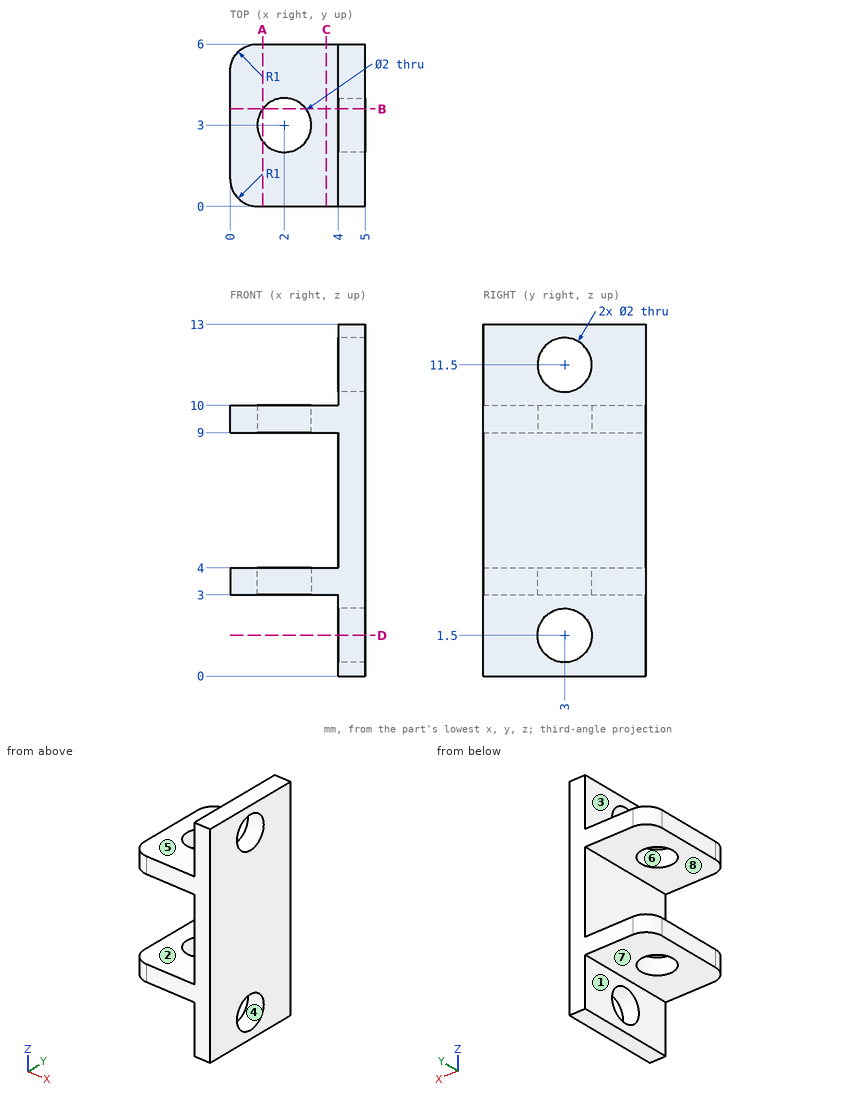
Geometry check sheet. Reference: drawing and pictorial views, mm from the part's lowest x, y, z. A direction names the side the tool comes from. Round coordinates to 2 decimals unless told otherwise and drop trailing zeros. Loops run counter-clockwise (first coordinate to the right, second up) from the corner with the lowest first, then second, coordinate; pieces in that order, holes last. Notation, with made-up numbers: (5, 71) - (23, 71) arc R11 ccw to (23, 76) - close; hole circle Ø1 at (22.25, 75.25). An arc over 180 degrees is marked (long way). Use a Markdown table: item, result. Add a question column.
1. Section check D-D, the plane z = 1.5. Record the boundary of the cut face in (x, y).
2. Release check for a two-part mould opening along Z. For the marked faces 5, 6, 7 and 8 record: released by +Z, released by -Z, zero draft, split by the parting line, or undercut.
3. Gauge pin test, flat ends, axial feed: pin 1 (2.5 mm diameter, centred on y = 2, z = 7, fed in from -X); pin 2 (0.9 mm diameter, centred on y = 3.5, z = 1.5, fed in from -X); pin 3 (2 mm diameter, centred on x = 2, y = 1.5, fed in from +Z); pin 4 (1.2 mm diameter, centred on x = 3, y = 3.5, fed in from -Z). Record the tip position at first contact, or that the pin passes through.
4. Thickness scan on probe 1 along Z at (x, y) = (4.5, 3); probe 2 along Y at (x, z) = (2, 9.8); probe 3 along Z at (x, y) = (0.8, 3.5). Record the ranges inside material, lowest first. Write a range as [from, to].
5. Section check C-C, the plane x = 3.55. Record the boundary of the cut face in (y, z).
6. Section check B-B, the plane y = 3.6. Record the boundary of the cut face in (x, z), plus the area to 3 significant figures.
7. Access from +Z, -Z, +X, -X, +Y, -Y to the whole of each face (thin tool, end or side, straight path). Record for the marked faces 1, 2, 3 and 4.
8. Section check A-A, the plane x = 1.2. Record the boundary of the cut face in (y, z), plus the area to 3 significant figures.
Checks:
| question | item | result |
|---|---|---|
| 1 | outline | (4, 0) - (5, 0) - (5, 2) - (4, 2) - close; (4, 4) - (5, 4) - (5, 6) - (4, 6) - close |
| 2 | face 5 | released by +Z |
| 2 | face 6 | zero draft |
| 2 | face 7 | released by -Z |
| 2 | face 8 | undercut |
| 3 | pin 1 | stops at x = 4 |
| 3 | pin 2 | passes through |
| 3 | pin 3 | stops at z = 10 |
| 3 | pin 4 | stops at z = 3 |
| 4 | probe 1 | z = [0, 0.5], [2.5, 10.5], [12.5, 13] |
| 4 | probe 2 | y = [0, 2], [4, 6] |
| 4 | probe 3 | z = [3, 4], [9, 10] |
| 5 | outline | (0, 3) - (6, 3) - (6, 4) - (0, 4) - close; (0, 9) - (6, 9) - (6, 10) - (0, 10) - close |
| 6 | outline | (0, 3) - (1.2, 3) - (1.2, 4) - (0, 4) - close; (0, 9) - (1.2, 9) - (1.2, 10) - (0, 10) - close; (2.8, 3) - (4, 3) - (4, 2.3) - (5, 2.3) - (5, 10.7) - (4, 10.7) - (4, 10) - (2.8, 10) - (2.8, 9) - (4, 9) - (4, 4) - (2.8, 4) - close; (4, 0) - (5, 0) - (5, 0.7) - (4, 0.7) - close; (4, 12.3) - (5, 12.3) - (5, 13) - (4, 13) - close |
| 6 | area | 14.6 mm^2 |
| 7 | face 1 | -Z, -X, +Y, -Y |
| 7 | face 2 | -X, +Y, -Y |
| 7 | face 3 | +Z, -X, +Y, -Y |
| 7 | face 4 | +X, -X |
| 8 | outline | (0, 3) - (2.4, 3) - (2.4, 4) - (0, 4) - close; (0, 9) - (2.4, 9) - (2.4, 10) - (0, 10) - close; (3.6, 3) - (6, 3) - (6, 4) - (3.6, 4) - close; (3.6, 9) - (6, 9) - (6, 10) - (3.6, 10) - close |
| 8 | area | 9.60 mm^2 |
